```python
from build123d import *

# Parameters (mm, degrees)
SKETCH1_R           = 1.5
EXTRUDE1_DEPTH      = 7
EXTRUDE1_DEPTH_BACK = 7


with BuildPart() as part:
    # Sketch1 → Extrude1 (new body, two sides)
    with BuildSketch(Plane.XY) as extrude1_sk:
        Polygon((0, 3.464101615), (-3, 1.732050808), (-3, -1.732050808), (0, -3.464101615), (3, -1.732050808), (3, 1.732050808), align=None)
        Circle(SKETCH1_R, mode=Mode.SUBTRACT)
    extrude(amount=EXTRUDE1_DEPTH)
    extrude(extrude1_sk.sketch, amount=-EXTRUDE1_DEPTH_BACK)


solid = part.part
```
Build history of the part. All positions in model axes, mm. Round coordinates to 2 decimals unless told otherwise and drop trailing zeros. Order: outer loops, then holes, each group sorted by start corner. A loop starts at its lowest first (then second) coordinate and runs counter-clockwise, first axis right, second up. Notation, with made-up numbers: (-13, 11.5) - (14, 11.5) arc R23 cw to (14, 28.5) - close; hole circle Ø6 at (-9, -28). An arc over 180 degrees is marked (long way). Use a Markdown table: item, result.
1) Saw through at D-D on y = 1. Write the cut outline in (x, z), and give its area (3 significant figures).
Recorded:
| item | result |
|---|---|
| outline | (-3, -7) - (-1.12, -7) - (-1.12, 7) - (-3, 7) - close; (1.12, -7) - (3, -7) - (3, 7) - (1.12, 7) - close |
| area | 52.7 mm² |
2) Flat gauge pins, fed straight in: pin 1 Ø1 at (x, z) = (-1.5, 2) entering from +Y; pin 2 Ø1 at (y, z) = (-2.5, 2) entering from -X; pin 3 Ø3 at (x, z) = (2, -1.5) entering from +Y. Where does each tip first touch, or does it go through?
Recorded:
| item | result |
|---|---|
| pin 1 | stops at y = 2.89 |
| pin 2 | stops at x = -2.54 |
| pin 3 | stops at y = 3.18 |
3) Saw through at C-C on x = 2.5. Write the cut outline in (y, z), and give its area (3 significant figures).
Recorded:
| item | result |
|---|---|
| outline | (-2.02, -7) - (2.02, -7) - (2.02, 7) - (-2.02, 7) - close |
| area | 56.6 mm² |
4) Saw through at A-A on z = 4.5. Write the cut outline in (x, y).
Recorded:
| item | result |
|---|---|
| outline | (-3, -1.73) - (0, -3.46) - (3, -1.73) - (3, 1.73) - (0, 3.46) - (-3, 1.73) - close; hole circle Ø3 at (0, 0) |
5) Pull direction X, two halves, no side cores. Call faces 1 (the face through (-1.5, 2.6, 0.1)), 2 (the face through (1.5, 2.6, 0.1)), 3 (the face through (-0.7, -1.5, -7)), 4 (the face through (-1.5, 0.07, -0.1)): pulls with the +X half, pulls with the -X half, needs draft (parallel to the pull), parting line crosses it, or undercut.
Recorded:
| item | result |
|---|---|
| face 1 | pulls with the -X half |
| face 2 | pulls with the +X half |
| face 3 | needs draft |
| face 4 | undercut |
6) Wall check: L1, parallel to Y at x = -0.5, z = -3.75; L2, parallel to X at y = 1, z = 3; L3, parallel to X at y = -1.25, z = 6.5. Give the ranges that are in metal, low to high.
Recorded:
| item | result |
|---|---|
| L1 | y = -3.18 to -1.41, 1.41 to 3.18 |
| L2 | x = -3 to -1.12, 1.12 to 3 |
| L3 | x = -3 to -0.83, 0.83 to 3 |
7) Saw through at B-B on y = 0. Write the cut outline in (x, z), and give its area (3 significant figures).
Recorded:
| item | result |
|---|---|
| outline | (-3, -7) - (-1.5, -7) - (-1.5, 7) - (-3, 7) - close; (1.5, -7) - (3, -7) - (3, 7) - (1.5, 7) - close |
| area | 42.0 mm² |
